Here's how the part is built. I have some questions about the finished solid (model axes, mm). Face numbers are marked on the shaded views. A direction names the side the tool comes from. Round coordinates to 2 decimals unless told otherwise and drop trailing zeros. Write each loop counter-clockwise with the first axis right and the second up, starting at its lowest first coordinate (ties: lowest second). Pieces come first, ordered by that corner, then holes. Notation, with made-up numbers: M -18.5,85.5 L -4.5,85.5 A11 cw -4.5,99.5 Z; hole C 11.25,81.5 d1. An arc over 180 degrees is marked long. Use one line per item in the form item = value. Start each with the question number.
Q1. I need wall thicknesses on line 1 along Z through (x, y) = (9, 172.5); line 2 along Y through (x, z) = (84, 88). Which ranges of each line are inside material? Lowest first, please. Write a range as from..to.
Q2. For the marked faces 1 and 2, which set-ups out of +Z, -Z, +X, -X, +Y, -Y let a thin tool reach every point of the face, with its end or its side?
Q3. I want a section at A-A on y = 41. List the corners of the cut face in (x, z) for me, and give its area (3 significant figures).
Q4. I want a section at C-C on x = 86.5. List the corners of the cut face in (y, z) for me, and give its area (3 significant figures).
Q5. I want a section at B-B on z = 69. List the corners of the cut face in (x, y) for me.
Q6. I'm going to push a flat-ended pin straight in: pin 1 Ø1 at (x, z) = (-27.5, 61) entering from +Y. Where does the tip first touch, or does it pass through?
Q7. We'd pull the mould along Z, two halves only. Please class the marked faces 3, 4, 5 and 6: +Z half, -Z half, draft (parallel to the pull), parting line (faces both ways), or undercut.
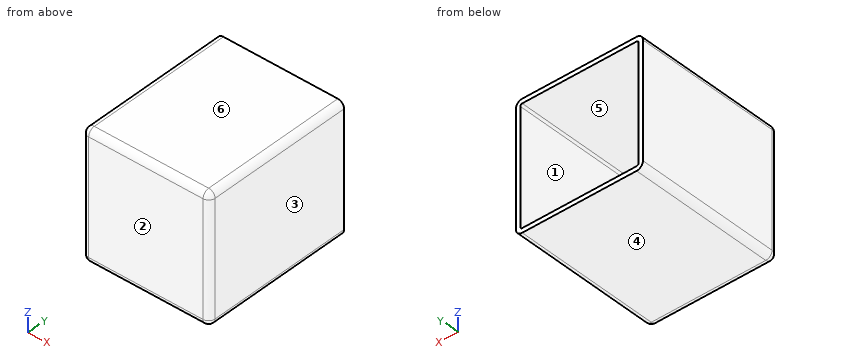
```python
from build123d import *

# Parameters (mm, degrees)
SKETCH1_W           = 200
SKETCH1_H           = 200
BOSS_EXTRUDE1_DEPTH = 240
FILLET1_R           = 10
SHELL1_T            = -7


with BuildPart() as part:
    # Sketch1 → Boss-Extrude1 (new body)
    with BuildSketch(Plane(origin=(0, 0, 0), x_dir=(1, 0, 0), z_dir=(0, 1, 0))):
        Rectangle(SKETCH1_W, SKETCH1_H)
    extrude(amount=BOSS_EXTRUDE1_DEPTH)

    # Fillet1
    fillet1_edges = [part.edges().sort_by_distance(p)[0] for p in [
        (0, 0, -100),
        (100, 0, 0),
        (0, 0, 100),
        (-100, 0, 0),
        (-100, 120, -100),
        (100, 120, -100),
        (100, 120, 100),
        (-100, 120, 100),
    ]]
    fillet(fillet1_edges, radius=FILLET1_R)

    # Shell1
    shell1_openings = [part.faces().sort_by_distance(p)[0] for p in [
        (0, 240, 0),
    ]]
    offset(amount=SHELL1_T, openings=shell1_openings, kind=Kind.INTERSECTION)


solid = part.part
```
Reported:
q1.line_1 = -100..-93, 93..100
q1.line_2 = 0..7
q2.face_1 = +Y
q2.face_2 = +Z, -Z, +X, -X, -Y
q3.outline = M -100,-90 A10 ccw -90,-100 L 90,-100 A10 ccw 100,-90 L 100,90 A10 ccw 90,100 L -90,100 A10 ccw -100,90 Z; hole M -93,-90 A3 ccw -90,-93 L 90,-93 A3 ccw 93,-90 L 93,90 A3 ccw 90,93 L -90,93 A3 ccw -93,90 Z
q3.area = 5,330 mm^2
q4.outline = M 0,-90 A10 ccw 10,-100 L 240,-100 L 240,-93 L 10,-93 A3 cw 7,-90 L 7,90 A3 cw 10,93 L 240,93 L 240,100 L 10,100 A10 ccw 0,90 Z
q4.area = 4,620 mm^2
q5.outline = M -100,10 A10 ccw -90,0 L 90,0 A10 ccw 100,10 L 100,240 L 93,240 L 93,10 A3 cw 90,7 L -90,7 A3 cw -93,10 L -93,240 L -100,240 Z
q6.pin_1 = 7
q7.face_3 = draft
q7.face_4 = -Z half
q7.face_5 = undercut
q7.face_6 = +Z half
